```python
from build123d import *

# Parameters (mm, degrees)
F0_R         = 60
F0_R_2       = 9
F1_DEPTH     = 0.15
F2_R         = 59
F1_FACE1_R   = 60
F1_FACE1_R_2 = 9
F3_DEPTH     = 0.25
F4_DEPTH     = 0.501


with BuildPart() as f1:
    # F0 (on Front) → F1 (new body, symmetric)
    with BuildSketch(Plane.XZ):
        Circle(F0_R)
        Circle(F0_R_2, mode=Mode.SUBTRACT)
    extrude(amount=F1_DEPTH, both=True)

    # F2 (on face) + F1_face1 (on face) → F3 (join, symmetric)
    with BuildSketch(Plane(origin=(0, 0.15, 0), x_dir=(-1, 0, 0), z_dir=(0, 1, 0))):
        Circle(F2_R)
    with BuildSketch(Plane.XZ.offset(0.15)):
        Circle(F1_FACE1_R)
        Circle(F1_FACE1_R_2, mode=Mode.SUBTRACT)
    extrude(amount=F3_DEPTH, both=True, dir=(0, 1, 0))

    # F4 (cut, through all): a face of the model
    f4_faces = [f1.faces().sort_by_distance(p)[0] for p in [
        (0, -0.1, 0),
    ]]
    extrude(f4_faces, amount=-F4_DEPTH, mode=Mode.SUBTRACT)


solid = f1.part
```
Model file for the job. Use its own axes, mm. A direction names the side the tool comes from. Give positions to 0.01 mm unless a question says otherwise; leave off trailing zeros. Loops run counter-clockwise (first coordinate to the right, second up) from the corner with the lowest first, then second, coordinate; pieces in that order, holes last. Notation, with made-up numbers: M 5,-8 L 46,-8 A30 cw 46,28 Z; hole C 57,80 d3. An arc over 180 degrees is marked long. Use one line per item in the form item = value.
Item 1: Slice it at D-D on x = -26. List the corners of the cut face in (y, z).
Filled in:
outline = M -0.4,-54.07 L 0.15,-54.07 L 0.15,-52.96 L 0.4,-52.96 L 0.4,52.96 L 0.15,52.96 L 0.15,54.07 L -0.4,54.07 Z
Item 2: Drill centre lines: L1, parallel to Z at x = 0, y = 0.25; L2, parallel to Z at x = 0, y = -0.15; L3, parallel to Z at x = -27.5, y = 0.1. Where is each one in solid material? Low to high.
Filled in:
L1 = -59 to -9, 9 to 59
L2 = -60 to -9, 9 to 60
L3 = -53.33 to 53.33
Item 3: Slice it at C-C on z = 33.5. List the corners of the cut face in (x, y).
Filled in:
outline = M -49.78,-0.4 L 49.78,-0.4 L 49.78,0.15 L 48.57,0.15 L 48.57,0.4 L -48.57,0.4 L -48.57,0.15 L -49.78,0.15 Z
Item 4: Slice it at A-A on z = 0. List the corners of the cut face in (x, y), and give its area (3 significant figures).
Filled in:
outline = M -60,-0.4 L -9,-0.4 L -9,0.4 L -59,0.4 L -59,0.15 L -60,0.15 Z; M 9,-0.4 L 60,-0.4 L 60,0.15 L 59,0.15 L 59,0.4 L 9,0.4 Z
area = 81.1 mm^2
Item 5: Slice it at B-B on x = 0. List the corners of the cut face in (y, z).
Filled in:
outline = M -0.4,-60 L 0.15,-60 L 0.15,-59 L 0.4,-59 L 0.4,-9 L -0.4,-9 Z; M -0.4,9 L 0.4,9 L 0.4,59 L 0.15,59 L 0.15,60 L -0.4,60 Z
Item 6: Which spindle directions (+Z, -Z, +X, -X, +Y, -Y) get a long thin tool onto all of the face, cutting with end or side? Do faces 1 (the flat face through (44, 0.15, -40)), 2 (the flat face through (1, 0.4, -12)). Say none if no direction does.
Filled in:
face_1 = +Y
face_2 = +Z, -Z, +X, -X, +Y
